```python
from build123d import *

# Parameters (mm, degrees)
SKETCH1_R                = 19.6
SKETCH1_R_2              = 16.6
BOSS_EXTRUDE1_DEPTH      = 20
SKETCH2_R                = 19.6
BOSS_EXTRUDE2_DEPTH      = 5
BOSS_EXTRUDE4_DEPTH      = 25
BOSS_EXTRUDE4_DEPTH_BACK = 25
SKETCH3_R                = 5.25
SKETCH4_R                = 39.6
SKETCH4_R_2              = 19.6
CUT_EXTRUDE_THIN1_DEPTH  = 25
CUT_EXTRUDE1_DEPTH       = 25
CUT_EXTRUDE1_DEPTH_BACK  = 25
SKETCH6_R                = 1.75


with BuildPart() as part:
    # Sketch1 → Boss-Extrude1 (new body)
    with BuildSketch(Plane(origin=(0, 0, 0), x_dir=(0, 1, 0), z_dir=(0, 0, 1))):
        with Locations(Location((0, 0, 0), (0, 0, 270))):
            Circle(SKETCH1_R)
        with Locations(Location((0, 0, 0), (0, 0, 270))):
            Circle(SKETCH1_R_2, mode=Mode.SUBTRACT)
    extrude(amount=BOSS_EXTRUDE1_DEPTH)

    # Sketch2 → Boss-Extrude2 (add)
    with BuildSketch(Plane.XY.offset(20)):
        Circle(SKETCH2_R)
    extrude(amount=BOSS_EXTRUDE2_DEPTH)

    # Sketch3 → Boss-Extrude4 (add, two sides: drawn at the far end of the back side and taken through both)
    with BuildSketch(Plane.YZ.offset(-BOSS_EXTRUDE4_DEPTH_BACK)):
        with BuildLine():
            Line((19.6, 25), (0, 25))
            Line((0, 25), (-19.6, 25))
            ThreePointArc((-19.6, 25), (0, 38.529292798), (19.6, 25))
        make_face()
        with Locations(Location((0, 31.139297983, 0), (0, 0, 270))):
            Circle(SKETCH3_R, mode=Mode.SUBTRACT)
    extrude(amount=BOSS_EXTRUDE4_DEPTH + BOSS_EXTRUDE4_DEPTH_BACK)

    # Sketch4 → Cut-Extrude-Thin1 (cut)
    with BuildSketch(Plane(origin=(0, 0, 20), x_dir=(1, 0, 0), z_dir=(0, 0, -1))):
        Circle(SKETCH4_R)
        Circle(SKETCH4_R_2, mode=Mode.SUBTRACT)
    extrude(amount=-CUT_EXTRUDE_THIN1_DEPTH, mode=Mode.SUBTRACT)

    # Sketch6 → Cut-Extrude1 (cut, two sides: drawn at the far end of the back side and taken through both)
    with BuildSketch(Plane.YZ.offset(-CUT_EXTRUDE1_DEPTH_BACK)):
        with Locations(Location((0, 9.747221623, 0), (0, 0, 90))):
            Circle(SKETCH6_R)
    extrude(amount=CUT_EXTRUDE1_DEPTH + CUT_EXTRUDE1_DEPTH_BACK, mode=Mode.SUBTRACT)


solid = part.part
```
The listing builds one solid part. Answer for the finished solid, in the listing's coordinates (mm). A direction names the side the tool comes from. Round coordinates to 2 decimals unless told otherwise and drop trailing zeros. Loops run counter-clockwise (first coordinate to the right, second up) from the corner with the lowest first, then second, coordinate; pieces in that order, holes last. Notation, with made-up numbers: (60, 58) -> (102, 58) arc R31 ccw to (102, 86) -> close; hole circle Ø2 at (41, 69.25). An arc over 180 degrees is marked (long way). Use one line per item in the form item = value.
1. Flat-ended cylindrical pins translate along their axes: pin 1 Ø1.5 at (x, y) = (-1, -13) entering from -Z; pin 2 Ø8 at (x, y) = (-4.5, -15.5) entering from +Z; pin 3 Ø4 at (y, z) = (13, 6) entering from -X. Find the tip coordinate at first contact, or state that the pin passes through.
Answer key:
pin_1 = 20
pin_2 = 35.09
pin_3 = -16.22
2. The part is cut by section A-A on x = -2.5. Determine the outline of the cut face in (y, z).
Answer key:
outline = (-19.44, 0) -> (-16.41, 0) -> (-16.41, 20) -> (16.41, 20) -> (16.41, 0) -> (19.44, 0) -> (19.44, 25.41) arc R20.96 ccw to (-19.44, 25.41) -> close; hole circle Ø10.5 at (0, 31.14)
3. A tool of negligible diameter and unlimited length cuts with its end or side. For faces 1 (the cylindrical face through (15.334, -6.358, 9.86)), 2 (the cylindrical face through (-0.28, -2.01, 26.29)), from which of +Z, -Z, +X, -X, +Y, -Y can it reach the whole face along a straight path? Write none if from no direction.
Answer key:
face_1 = -Z
face_2 = +X, -X
4. Find the intervals of material crossed by probe 1 along Z at (x, y) = (17.85, 0); probe 2 along X at (y, z) = (0.5, 8); probe 3 along Y at (x, z) = (0, 9.5), in increasing order. Write a range as [from, to].
Answer key:
probe_1 = [0, 8], [11.5, 25.89], [36.39, 38.53]
probe_2 = [-19.59, -16.59], [16.59, 19.59]
probe_3 = [-19.6, -16.6], [16.6, 19.6]
5. The part is cut by section D-D on y = 10. Determine the outline of the cut face in (x, z), and give its area (3 significant figures).
Answer key:
outline = (-16.86, 0) -> (-13.25, 0) -> (-13.25, 20) -> (13.25, 20) -> (13.25, 0) -> (16.86, 0) -> (16.86, 35.99) -> (-16.86, 35.99) -> close
area = 683 mm²
6. For a pull along X with two mould halves and no side action, classify faces 3 (the flat face through (0, 0, 20)), 4 (the flat face through (-15, 9, 0)) as released by +X, released by -X, zero draft, split by the parting line, or undercut.
Answer key:
face_3 = undercut
face_4 = zero draft
7. The part is cut by section B-B on y = -7. Determine the outline of the cut face in (x, z).
Answer key:
outline = (-18.31, 0) -> (-15.05, 0) -> (-15.05, 20) -> (15.05, 20) -> (15.05, 0) -> (18.31, 0) -> (18.31, 37.33) -> (-18.31, 37.33) -> close
8. The part is cut by section C-C on z = 16. Determine the outline of the cut face in (x, y).
Answer key:
outline = circle Ø39.2 at (0, 0); hole circle Ø33.2 at (0, 0)
